Check sheet for the modelled part. Datum: model origin and axes. Units: mm. Face numbers are marked on the shaded views. Coordinates: 2 decimals unless noted, no trailing zeros. Loops run counter-clockwise (first coordinate to the right, second up) from the corner with the lowest first, then second, coordinate; pieces in that order, holes last. Notation, with made-up numbers: M 56,80.5 L 74,80.5 A20 cw 74,87.5 Z; hole C -29,18 d7. An arc over 180 degrees is marked long. Write each question's results on one line, items separated by ' | '. Start each with the question number.
from build123d import *

# Parameters (mm, degrees)
F1_DEPTH = 5
F3_DEPTH = 5
F4_DEPTH = 70
F5_W     = 16.032818
F5_H     = 10
F6_DEPTH = 5


with BuildPart() as f1:
    # F0 (on Right) → F1 (new body)
    with BuildSketch(Plane.YZ):
        Polygon((-7.5, 0), (0, 0), (7.5, 0), (7.5, 10), (-7.5, 10), align=None)
    extrude(amount=F1_DEPTH)

    # F2 (on face) → F3 (join)
    with BuildSketch(Plane.YZ.offset(5)):
        Polygon((7.532818, 6.2145), (8.532818, 6.2145), (8.532818, 10), (7.5, 10), (7.5, 6.268203), align=None)
        Polygon((7.5, 6.194444), (7.5, 0), (8.532818, 0), (8.532818, 6.2145), (7.532818, 6.2145), align=None)
    extrude(amount=-F3_DEPTH)

    # F2 (on face) → F4 (join)
    with BuildSketch(Plane.YZ.offset(5)):
        Polygon((-7.5, 0), (0, 0), (0, 1), (-1, 1), (-6.5, 1), (-6.5, 9), (-5.888889, 9), (-6.5, 10), (-7.5, 10), align=None)
        Polygon((-6.5, 1), (-1, 1), (-5.888889, 9), (-6.5, 9), align=None)
        Polygon((-1, 1), (0, 1), (6.5, 1), (6.5, 5.583333), align=None)
        Polygon((7.5, 6.194444), (7.5, 0), (8.532818, 0), (8.532818, 6.2145), (7.532818, 6.2145), align=None)
        Polygon((0, 1), (0, 0), (7.5, 0), (7.5, 6.194444), (6.5, 5.583333), (6.5, 1), align=None)
        Polygon((7.532818, 6.2145), (8.532818, 6.2145), (8.532818, 10), (7.5, 10), (7.5, 6.268203), align=None)
        Polygon((5.219457, 10), (7.5, 6.268203), (7.5, 10), align=None)
    extrude(amount=F4_DEPTH)

    # F5 (on face) → F6 (join)
    with BuildSketch(Plane.YZ.offset(75)):
        with Locations((0.516409, 5)):
            Rectangle(F5_W, F5_H)
        Polygon((-7.5, 10), (-7.5, 0), (8.532818, 0), (8.532818, 10), (-6.5, 10), align=None)
    extrude(amount=F6_DEPTH)


with BuildPart() as f1_1:
    # F7: moved
    add(f1.part.moved(Location((-40, 0, 0))))


solid = f1_1.part
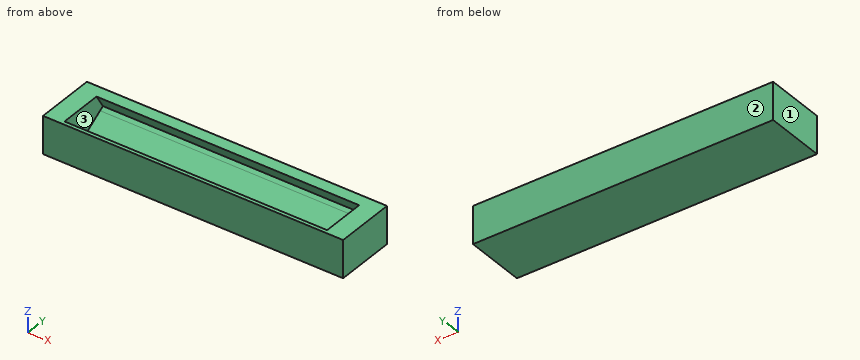
1) Section check A-A (z = 3.5). Enter the section's corners in (x, y), then the cut area to 3 significant figures.
2) Gauge pin test, flat end, axial feed: P1, Ø4, axis at x = 1.5, y = 1.5, coming from the +Z side. Record the tip position at first contact, or that the pin passes through.
3) Section check C-C (y = 0). Enter the section's corners in (x, z), then the cut area to 3 significant figures.
4) Release check for a two-part mould opening along Y. For the marked faces 1, 2 and 3 record: +Y half, -Y half, draft (parallel to the pull), parting line (faces both ways), or undercut.
5) Section check D-D (y = 4.5). Enter the section's corners in (x, z), then the cut area to 3 significant figures.
6) Thickness scan on probe 1 along X at (y, z) = (-1.75, 3); probe 2 along Y at (x, z) = (18.5, 6.25); probe 3 along Z at (x, y) = (16, -5). Record the ranges inside material, lowest first.
Return value:
1) outline: M -40,-7.5 L 40,-7.5 L 40,8.53 L -40,8.53 Z; hole M -35,-2.53 L 35,-2.53 L 35,3.09 L -35,3.09 Z | area: 889 mm2
2) P1: stops at z = 3.75
3) outline: M -40,0 L 40,0 L 40,10 L 35,10 L 35,1.61 L -35,1.61 L -35,10 L -40,10 Z | area: 213 mm2
4) face 1: draft | face 2: +Y half | face 3: undercut
5) outline: M -40,0 L 40,0 L 40,10 L 35,10 L 35,4.36 L -35,4.36 L -35,10 L -40,10 Z | area: 405 mm2
6) probe 1: x = -40 to -35, 35 to 40 | probe 2: y = -7.5 to -4.21, 7.51 to 8.53 | probe 3: z = 0 to 7.55
